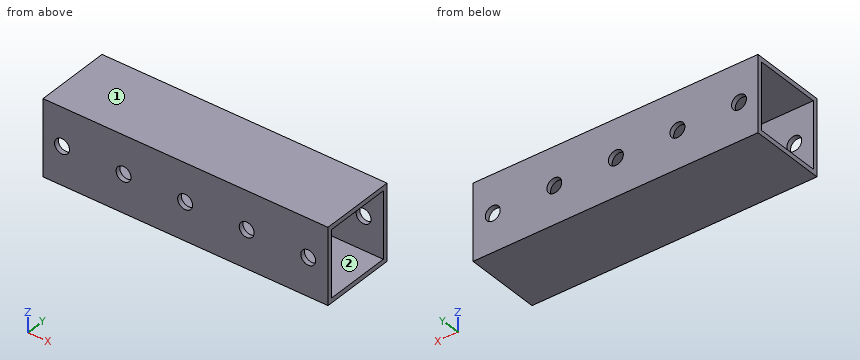
from build123d import *

# Parameters (mm, degrees)
SKETCH1_W           = 25.4
SKETCH1_H           = 25.4
SKETCH1_W_2         = 22.225
SKETCH1_H_2         = 22.225
BOSS_EXTRUDE1_DEPTH = 95.25
SKETCH2_R           = 2.4892
CUT_EXTRUDE1_DEPTH  = 95.25


with BuildPart() as part:
    # Sketch1 → Boss-Extrude1 (new body)
    with BuildSketch(Plane(origin=(0, 0, 0), x_dir=(0, 0, -1), z_dir=(1, 0, 0))):
        with Locations((12.7, 12.7)):
            Rectangle(SKETCH1_W, SKETCH1_H)
        with Locations((12.7, 12.7)):
            Rectangle(SKETCH1_W_2, SKETCH1_H_2, mode=Mode.SUBTRACT)
    extrude(amount=BOSS_EXTRUDE1_DEPTH)

    # Sketch2 → Cut-Extrude1 (cut)
    with BuildSketch(Plane(origin=(0, 25.4, 0), x_dir=(1, 0, 0), z_dir=(0, 1, 0))):
        with Locations(Location((6.35, 12.7, 0), (0, 0, 270))):
            Circle(SKETCH2_R)
        with Locations(Location((26.924, 12.7, 0), (0, 0, 270))):
            Circle(SKETCH2_R)
        with Locations(Location((47.498, 12.7, 0), (0, 0, 270))):
            Circle(SKETCH2_R)
        with Locations(Location((68.072, 12.7, 0), (0, 0, 270))):
            Circle(SKETCH2_R)
        with Locations(Location((88.646, 12.7, 0), (0, 0, 270))):
            Circle(SKETCH2_R)
    extrude(amount=-CUT_EXTRUDE1_DEPTH, mode=Mode.SUBTRACT)


solid = part.part
The model under review builds one solid part; all positions refer to its coordinate system, in mm. Face numbers are marked on the shaded views. A direction names the side the tool comes from. Round coordinates to 2 decimals unless told otherwise and drop trailing zeros. Loops run counter-clockwise (first coordinate to the right, second up) from the corner with the lowest first, then second, coordinate; pieces in that order, holes last. Notation, with made-up numbers: (-2, 54) -> (2, 54) arc R35 cw to (2, 92) -> close; hole circle Ø8 at (53.5, -14.5). An arc over 180 degrees is marked (long way). Write item = value, one per line. Start each with the question number.
Item 1: Take a section at C-C on x = 6.35. Give the boundary of the cut face in (y, z).
Item 2: Take a section at B-B on z = -21.5. Give the boundary of the cut face in (x, y), plus the area to 3 significant figures.
Item 3: To check wall thickness, follow L1, parallel to X at y = 24.5, z = -12.7; L2, parallel to Z at x = 5, y = 5; L3, parallel to Y at x = 31, z = -5.25. State the ranges of each line that lie inside material, in increasing order.
Item 4: For the marked faces 1 and 2, list the 3-axis set-ups (+Z, -Z, +X, -X, +Y, -Y) from which the entire face can be reached by the end or side of a thin tool; tool diameter is ignored.
Item 5: Take a section at D-D on x = 40. Give the boundary of the cut face in (y, z).
Item 6: Take a section at A-A on y = 21. Give the boundary of the cut face in (x, z).
Result:
q1.outline = (0, -25.4) -> (25.4, -25.4) -> (25.4, -15.19) -> (23.81, -15.19) -> (23.81, -23.81) -> (1.59, -23.81) -> (1.59, -15.19) -> (0, -15.19) -> close; (0, -10.21) -> (1.59, -10.21) -> (1.59, -1.59) -> (23.81, -1.59) -> (23.81, -10.21) -> (25.4, -10.21) -> (25.4, 0) -> (0, 0) -> close
q2.outline = (0, 0) -> (95.25, 0) -> (95.25, 1.59) -> (0, 1.59) -> close; (0, 23.81) -> (95.25, 23.81) -> (95.25, 25.4) -> (0, 25.4) -> close
q2.area = 302 mm²
q3.L1 = 0 to 3.86, 8.84 to 24.43, 29.41 to 45.01, 49.99 to 65.58, 70.56 to 86.16, 91.14 to 95.25
q3.L2 = -25.4 to -23.81, -1.59 to 0
q3.L3 = 0 to 1.59, 23.81 to 25.4
q4.face_1 = +Z, +X, -X, +Y, -Y
q4.face_2 = +X, -X
q5.outline = (0, -25.4) -> (25.4, -25.4) -> (25.4, 0) -> (0, 0) -> close; hole (1.59, -23.81) -> (23.81, -23.81) -> (23.81, -1.59) -> (1.59, -1.59) -> close
q6.outline = (0, -25.4) -> (95.25, -25.4) -> (95.25, -23.81) -> (0, -23.81) -> close; (0, -1.59) -> (95.25, -1.59) -> (95.25, 0) -> (0, 0) -> close
